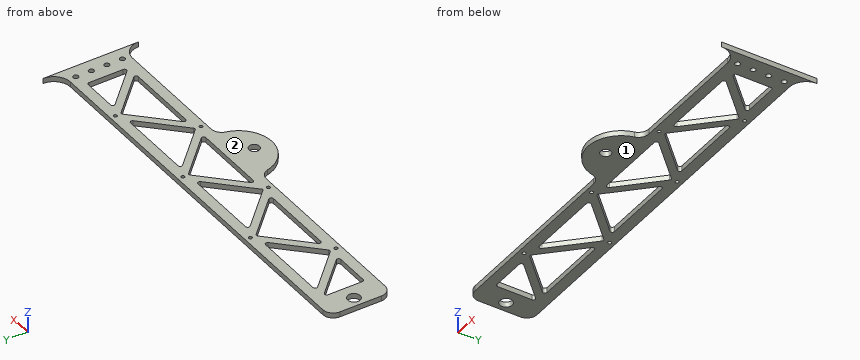
from build123d import *

# Parameters (mm, degrees)
BOSS_EXTRUDE1_DEPTH        = 5
CUT_EXTRUDE2_DEPTH         = 5
CUT_EXTRUDE3_REACH         = 7
FILLET1_R                  = 2
M6X1_0_TAPPED_HOLE1_D      = 5
M4X0_7_TAPPED_HOLE1_D      = 3.3
BOSS_EXTRUDE2_DEPTH        = 5
FILLET2_R                  = 10
F_10_0MM_DOWEL_HOLE1_D     = 10
BOSS_EXTRUDE3_DEPTH        = 5
F_12_0MM_DOWEL_HOLE1_D     = 12
F_12_0MM_DOWEL_HOLE1_DEPTH = 5


with BuildPart() as part:
    # Sketch1 → Boss-Extrude1 (new body)
    with BuildSketch(Plane.XY):
        with BuildLine():
            Line((-10, 0), (-390, 0))
            ThreePointArc((-390, 0), (-397.071067812, 2.928932188), (-400, 10))
            Line((-400, 10), (-400, 50))
            ThreePointArc((-400, 50), (-397.071067812, 57.071067812), (-390, 60))
            Line((-390, 60), (-10, 60))
            ThreePointArc((-10, 60), (-2.928932188, 57.071067812), (0, 50))
            Line((0, 50), (0, 10))
            ThreePointArc((0, 10), (-2.928932188, 2.928932188), (-10, 0))
        make_face()
    extrude(amount=BOSS_EXTRUDE1_DEPTH)

    # Sketch2 → Cut-Extrude2 (cut)
    with BuildSketch(Plane.XY.offset(5)):
        Polygon((-375, 10), (-365, 10), (-365, 40), (-375, 50), align=None)
        Polygon((-365, 40), (-365, 10), (-355, 10), (-355, 30), align=None)
        Polygon((-355, 30), (-355, 10), (-345, 10), (-345, 20), align=None)
        Polygon((-345, 20), (-345, 10), (-335, 10), align=None)
        Polygon((-305, 20), (-315, 10), (-305, 10), align=None)
        Polygon((-305, 20), (-305, 10), (-295, 10), (-295, 30), align=None)
        Polygon((-295, 30), (-295, 10), (-285, 10), (-285, 40), align=None)
        Polygon((-285, 40), (-285, 10), (-275, 10), (-275, 50), align=None)
        Polygon((-275, 50), (-275, 10), (-265, 10), (-265, 40), align=None)
        Polygon((-265, 40), (-265, 10), (-255, 10), (-255, 30), align=None)
        Polygon((-255, 30), (-255, 10), (-245, 10), (-245, 20), align=None)
        Polygon((-245, 20), (-245, 10), (-235, 10), align=None)
        Polygon((-205, 20), (-215, 10), (-205, 10), align=None)
        Polygon((-205, 20), (-205, 10), (-195, 10), (-195, 30), align=None)
        Polygon((-195, 30), (-195, 10), (-185, 10), (-185, 40), align=None)
        Polygon((-185, 40), (-185, 10), (-175, 10), (-175, 50), align=None)
        Polygon((-175, 50), (-175, 10), (-165, 10), (-165, 40), align=None)
        Polygon((-165, 40), (-165, 10), (-155, 10), (-155, 30), align=None)
        Polygon((-155, 30), (-155, 10), (-145, 10), (-145, 20), align=None)
        Polygon((-145, 20), (-145, 10), (-135, 10), align=None)
        Polygon((-45, 20), (-45, 10), (-35, 10), align=None)
        Polygon((-55, 30), (-55, 10), (-45, 10), (-45, 20), align=None)
        Polygon((-65, 40), (-65, 10), (-55, 10), (-55, 30), align=None)
        Polygon((-75, 50), (-75, 10), (-65, 10), (-65, 40), align=None)
        Polygon((-85, 40), (-85, 10), (-75, 10), (-75, 50), align=None)
        Polygon((-95, 30), (-95, 10), (-85, 10), (-85, 40), align=None)
        Polygon((-105, 20), (-105, 10), (-95, 10), (-95, 30), align=None)
        Polygon((-105, 20), (-115, 10), (-105, 10), align=None)
        Polygon((-25, 50), (-35, 50), (-35, 20), (-25, 10), align=None)
        Polygon((-35, 50), (-45, 50), (-45, 30), (-35, 20), align=None)
        Polygon((-45, 50), (-55, 50), (-55, 40), (-45, 30), align=None)
        Polygon((-55, 50), (-65, 50), (-55, 40), align=None)
    extrude(amount=-CUT_EXTRUDE2_DEPTH, mode=Mode.SUBTRACT)

    # Sketch3 → Cut-Extrude3 (cut, up to next)
    with BuildSketch(Plane.XY.offset(5), mode=Mode.PRIVATE) as cut_extrude3_sk1:
        Polygon((-365, 50), (-285, 50), (-325, 10), align=None)
    cut_extrude3_tool1 = extrude(cut_extrude3_sk1.sketch, amount=-CUT_EXTRUDE3_REACH, mode=Mode.PRIVATE) & part.part
    add(cut_extrude3_tool1.solids().sort_by_distance((-325, 36.666667, 5))[0], mode=Mode.SUBTRACT)
    # Sketch3 → Cut-Extrude3 (cut, up to next)
    with BuildSketch(Plane.XY.offset(5), mode=Mode.PRIVATE) as cut_extrude3_sk2:
        Polygon((-225, 10), (-265, 50), (-185, 50), align=None)
    cut_extrude3_tool2 = extrude(cut_extrude3_sk2.sketch, amount=-CUT_EXTRUDE3_REACH, mode=Mode.PRIVATE) & part.part
    add(cut_extrude3_tool2.solids().sort_by_distance((-225, 36.666667, 5))[0], mode=Mode.SUBTRACT)
    # Sketch3 → Cut-Extrude3 (cut, up to next)
    with BuildSketch(Plane.XY.offset(5), mode=Mode.PRIVATE) as cut_extrude3_sk3:
        Polygon((-125, 10), (-165, 50), (-85, 50), align=None)
    cut_extrude3_tool3 = extrude(cut_extrude3_sk3.sketch, amount=-CUT_EXTRUDE3_REACH, mode=Mode.PRIVATE) & part.part
    add(cut_extrude3_tool3.solids().sort_by_distance((-125, 36.666667, 5))[0], mode=Mode.SUBTRACT)

    # Fillet1
    fillet1_edges = [part.edges().sort_by_distance(p)[0] for p in [
        (-325, 10, 2.5),
        (-365, 50, 2.5),
        (-285, 50, 2.5),
        (-265, 50, 2.5),
        (-185, 50, 2.5),
        (-165, 50, 2.5),
        (-85, 50, 2.5),
        (-125, 10, 2.5),
        (-375, 50, 2.5),
        (-335, 10, 2.5),
        (-375, 10, 2.5),
        (-315, 10, 2.5),
        (-275, 50, 2.5),
        (-235, 10, 2.5),
        (-215, 10, 2.5),
        (-175, 50, 2.5),
        (-135, 10, 2.5),
        (-65, 50, 2.5),
        (-25, 50, 2.5),
        (-25, 10, 2.5),
        (-75, 50, 2.5),
        (-35, 10, 2.5),
        (-115, 10, 2.5),
    ]]
    fillet(fillet1_edges, radius=FILLET1_R)

    # M6x1.0 Tapped Hole1 (through all)
    with Locations(Plane.XY.offset(5)):
        with Locations((-12.5, 52.5), (-12.5, 37.5), (-12.5, 22.5), (-12.5, 7.5)):
            Hole(M6X1_0_TAPPED_HOLE1_D / 2)

    # M4x0.7 Tapped Hole1 (through all)
    with Locations(Plane.XY.offset(5)):
        with Locations((-225, 5), (-175, 55), (-125, 5), (-75, 55), (-275, 55), (-325, 5)):
            Hole(M4X0_7_TAPPED_HOLE1_D / 2)

    # Sketch9 → Boss-Extrude2 (add)
    with BuildSketch(Plane.XY.offset(5)):
        with BuildLine():
            Line((-205.342623586, 0), (-141.342623586, 0))
            ThreePointArc((-141.342623586, 0), (-173.342623586, -32), (-205.342623586, 0))
        make_face()
    extrude(amount=-BOSS_EXTRUDE2_DEPTH)

    # Fillet2
    fillet2_edges = [part.edges().sort_by_distance(p)[0] for p in [
        (-205.342623586, 0, 2.5),
        (-141.342623586, 0, 2.5),
    ]]
    fillet(fillet2_edges, radius=FILLET2_R)

    # Ø10.0mm Dowel Hole1 (through all)
    with Locations(Plane.XY.offset(5)):
        with Locations((-173.342623586, -15)):
            Hole(F_10_0MM_DOWEL_HOLE1_D / 2)

    # Sketch12 → Boss-Extrude3 (add)
    with BuildSketch(Plane.XY.offset(5)):
        with BuildLine():
            Line((0, 76), (0, 50))
            ThreePointArc((0, 50), (-6.566018868, 57.294369811), (-16, 60))
            ThreePointArc((-16, 60), (-4.686291501, 64.686291501), (0, 76))
        make_face()
        with BuildLine():
            Line((0, 10), (0, -16))
            ThreePointArc((0, -16), (-4.686291501, -4.686291501), (-16, 0))
            ThreePointArc((-16, 0), (-6.566018868, 2.705630189), (0, 10))
        make_face()
    extrude(amount=-BOSS_EXTRUDE3_DEPTH)

    # Ø12.0mm Dowel Hole1
    with Locations(Plane.XY.offset(5)):
        with Locations((-390, 30)):
            Hole(F_12_0MM_DOWEL_HOLE1_D / 2, depth=F_12_0MM_DOWEL_HOLE1_DEPTH)


solid = part.part
The listing builds one solid part. Answer for the finished solid, in the listing's coordinates (mm). Face numbers are marked on the shaded views. Give positions to 0.01 mm unless a question says otherwise; leave off trailing zeros. Write each loop counter-clockwise with the first axis right and the second up, starting at its lowest first coordinate (ties: lowest second). Pieces come first, ordered by that corner, then holes.
Item 1: Section B-B, the plane z = 2.8 is taken. Count the separate pieces of the cut face and the enclosed holes in it, plus the area to 3 significant figures.
Item 2: Flat-ended cylindrical pins translate along their axes: P1, Ø3, axis at x = -276.5, y = 45.5, coming from the +Z side; P2, Ø1.5, axis at x = -84.5, z = 1.5, coming from the -Y side. Find the tip coordinate at first contact, or state that the pin passes through.
Item 3: Section A-A, the plane x = -349 is taken. Write down the section's boundary in (y, z).
Item 4: Find the intervals of material crossed by line 1 along Y through (x, z) = (-225, 3.7); line 2 along Y through (x, z) = (-275, 2.45); line 3 along Y through (x, z) = (-12.5, 1.4), in increasing order.
Item 5: Determine the mould class of the marked faces 1 and 2 for opening direction Z: released by +Z, released by -Z, zero draft, split by the parting line, or undercut.
Completed:
1. separate pieces: 1
1. enclosed holes: 20
1. area: 14,300 mm2
2. P1: passes through
2. P2: stops at y = 0
3. outline: (0, 0) - (10, 0) - (10, 5) - (0, 5) - close; (24, 0) - (34, 0) - (34, 5) - (24, 5) - close; (50, 0) - (60, 0) - (60, 5) - (50, 5) - close
4. line 1: y = 0 to 3.35, 6.65 to 10, 50 to 60
4. line 2: y = 0 to 10, 49.17 to 53.35, 56.65 to 60
4. line 3: y = -0.39 to 5, 10 to 20, 25 to 35, 40 to 50, 55 to 60.39
5. face 1: released by -Z
5. face 2: released by +Z
